Input: part model. Units: mm. Frame: model coordinates. A direction names the side the tool comes from. Round coordinates to 2 decimals unless told otherwise and drop trailing zeros. Write each loop counter-clockwise with the first axis right and the second up, starting at its lowest first coordinate (ties: lowest second). Pieces come first, ordered by that corner, then holes. Notation, with made-up numbers: M -5,60.25 L 19,60.25 A12 ccw 19,70.25 Z; hole C -21.75,-23.75 d1. An arc over 180 degrees is marked long. Answer as CSV lines item,"result". Start each with the question number.
```python
from build123d import *

# Parameters (mm, degrees)
BOSS_EXTRU_1_DEPTH           = 24.7
ENL_V_MAT_EXTRU_1_DEPTH      = 27.583688608
ENL_V_MAT_EXTRU_1_DEPTH_BACK = 27.583688608
D_GAGEMENT_M31_D             = 3
ESQUISSE5_W                  = 6
ESQUISSE5_H                  = 4.8
BOSS_EXTRU_2_DEPTH           = 1.3
ESQUISSE6_R                  = 1.4
BOSS_EXTRU_3_DEPTH           = 8
ESQUISSE7_W                  = 2
ESQUISSE7_H                  = 1
ENL_V_MAT_EXTRU_2_DEPTH      = 0.2


with BuildPart() as part:
    # Esquisse1 → Boss.-Extru.1 (new body)
    with BuildSketch(Plane.XY):
        with BuildLine():
            Line((-3.95, 5.05), (-3.95, 0))
            Line((-3.95, 0), (3.95, 0))
            Line((3.95, 0), (3.95, 5.05))
            ThreePointArc((3.95, 5.05), (0, 9), (-3.95, 5.05))
        make_face()
    extrude(amount=-BOSS_EXTRU_1_DEPTH)

    # Esquisse2 → Enlèv. mat.-Extru.1 (cut, two sides: drawn at the far end of the back side and taken through both)
    with BuildSketch(Plane(origin=(0, 0, 0), x_dir=(0, 0, -1), z_dir=(1, 0, 0)).offset(-ENL_V_MAT_EXTRU_1_DEPTH_BACK)):
        Polygon((6.9, 9), (8.9, 5.7), (24.7, 5.7), (24.7, 9), align=None)
    extrude(amount=ENL_V_MAT_EXTRU_1_DEPTH + ENL_V_MAT_EXTRU_1_DEPTH_BACK, mode=Mode.SUBTRACT)

    # Dégagement M31 (through all)
    with Locations(Plane(origin=(0, 5.7, 0), x_dir=(1, 0, 0), z_dir=(0, 1, 0))):
        with Locations((0, 19)):
            Hole(D_GAGEMENT_M31_D / 2)

    # Esquisse5 → Boss.-Extru.2 (add)
    with BuildSketch(Plane(origin=(0, 0, -24.7), x_dir=(-1, 0, 0), z_dir=(0, 0, -1))):
        with Locations((0, 2.4)):
            Rectangle(ESQUISSE5_W, ESQUISSE5_H)
    extrude(amount=BOSS_EXTRU_2_DEPTH)

    # Esquisse6 → Boss.-Extru.3 (add)
    with BuildSketch(Plane(origin=(0, 0, -26), x_dir=(-1, 0, 0), z_dir=(0, 0, -1))):
        with Locations((0, 3)):
            Circle(ESQUISSE6_R)
    extrude(amount=BOSS_EXTRU_3_DEPTH)

    # Esquisse7 → Enlèv. mat.-Extru.2 (cut)
    with BuildSketch(Plane(origin=(0, 5.7, 0), x_dir=(1, 0, 0), z_dir=(0, 1, 0))):
        with Locations((0, 12)):
            Rectangle(ESQUISSE7_W, ESQUISSE7_H)
    extrude(amount=-ENL_V_MAT_EXTRU_2_DEPTH, mode=Mode.SUBTRACT)


solid = part.part
```
Item 1: Line query: line 1 (X direction, y = 3.1, z = -19); line 2 (Z direction, x = 0, y = 1.9); line 3 (Z direction, x = 0, y = 4.5). Output: solid intervals per line, ascending. Write a range as [from, to].
Item 2: Access query for faces 5 (the face through (3, 2, -25)), 6 (the face through (0.303, 1.633, -29.944)), 7 (the face through (0, 4.8, -25)). Directions: +Z, -Z, +X, -X, +Y, -Y. A direction counts if a zero-diameter tool reaches every point of the face in a straight line with its end or side. Return the directions, or none.
Item 3: Draft query along Z for faces 1 (the face through (0, 5, 0)), 2 (the face through (0, 0, -13)), 3 (the face through (0.195, 2.81, -20.487)), 4 (the face through (0, 1, -26)). Return one class per face: +Z half, -Z half, draft (parallel to the pull), parting line (faces both ways), or undercut.
Item 4: Cut plane B-B, the plane x = 0. Return loops of the section in (y, z), plus the area to 3 significant figures.
Item 5: Cut plane C-C, the plane y = 3. Return loops of the section in (x, z), plus the area to 3 significant figures.
Item 6: Cut plane D-D, the plane x = -2.25. Return loops of the section in (y, z).
Item 7: Pin query (flat end, axial travel): pin 1 Ø1.5 at (x, y) = (-0.5, 6) entering from -Z; pin 2 Ø0.7 at (y, z) = (2.5, -25.5) entering from -X; pin 3 Ø0.5 at (x, z) = (0, -12) entering from +Y. Return the tip coordinate at first contact, or that it passes through.
Item 8: Cut plane A-A, the plane z = -19. Return loops of the section in (x, y).
Results list:
1,line 1,"[-3.95, -1.5], [1.5, 3.95]"
1,line 2,"[-34, -20.5], [-17.5, 0]"
1,line 3,"[-26, -20.5], [-17.5, 0]"
2,face 5,"-Z, +X, +Y, -Y"
2,face 6,"-Z"
2,face 7,"-Z, +X, -X, +Y"
3,face 1,"+Z half"
3,face 2,"draft"
3,face 3,"undercut"
3,face 4,"-Z half"
4,outline,"M 0,-26 L 1.6,-26 L 1.6,-34 L 4.4,-34 L 4.4,-26 L 4.8,-26 L 4.8,-24.7 L 5.7,-24.7 L 5.7,-20.5 L 0,-20.5 Z; M 0,-17.5 L 5.7,-17.5 L 5.7,-12.5 L 5.5,-12.5 L 5.5,-11.5 L 5.7,-11.5 L 5.7,-8.9 L 9,-6.9 L 9,0 L 0,0 Z"
4,area,"178 mm²"
5,outline,"M -3.95,-24.7 L -3,-24.7 L -3,-26 L -1.4,-26 L -1.4,-34 L 1.4,-34 L 1.4,-26 L 3,-26 L 3,-24.7 L 3.95,-24.7 L 3.95,0 L -3.95,0 Z; hole C 0,-19 d3"
5,area,"218 mm²"
6,outline,"M 0,-26 L 4.8,-26 L 4.8,-24.7 L 5.7,-24.7 L 5.7,-8.9 L 8.3,-7.33 L 8.3,0 L 0,0 Z"
7,pin 1,"z = -24.7"
7,pin 2,"x = -3"
7,pin 3,"y = 5.5"
8,outline,"M -3.95,0 L -1.5,0 L -1.5,5.7 L -3.9,5.7 A3.95 ccw -3.95,5.05 Z; M 1.5,0 L 3.95,0 L 3.95,5.05 A3.95 ccw 3.9,5.7 L 1.5,5.7 Z"
